```python
from build123d import *

# Parameters (mm, degrees)
BOSS_EXTRUDE1_DEPTH = 3.175
SKETCH2_R           = 2.159
CUT_EXTRUDE1_DEPTH  = 38.162422217
CUT_EXTRUDE2_DEPTH  = 38.162422217
FILLET1_R           = 6.35
FILLET2_R           = 1.905


with BuildPart() as part:
    # Sketch1 → Boss-Extrude1 (new body)
    with BuildSketch(Plane(origin=(0, 0, 0), x_dir=(1, 0, 0), z_dir=(0, 1, 0))):
        Polygon((-17.4625, 31.75), (0, 22.225), (17.4625, 31.75), (19.05, 3.175), (0, -19.05), (-19.05, 3.175), align=None)
    extrude(amount=BOSS_EXTRUDE1_DEPTH)

    # Sketch2 → Cut-Extrude1 (cut, through all)
    with BuildSketch(Plane(origin=(0, 3.175, 0), x_dir=(1, 0, 0), z_dir=(0, 1, 0))):
        with Locations(Location((0, -10.4775, 0), (0, 0, 270))):
            Circle(SKETCH2_R)
        with Locations(Location((-12.7, 3.4925, 0), (0, 0, 270))):
            Circle(SKETCH2_R)
        with Locations(Location((12.7, 3.4925, 0), (0, 0, 270))):
            Circle(SKETCH2_R)
        with Locations(Location((-12.7, 22.5425, 0), (0, 0, 270))):
            Circle(SKETCH2_R)
        with Locations(Location((12.7, 22.5425, 0), (0, 0, 270))):
            Circle(SKETCH2_R)
    extrude(amount=-CUT_EXTRUDE1_DEPTH, mode=Mode.SUBTRACT)

    # Sketch3 → Cut-Extrude2 (cut, through all)
    with BuildSketch(Plane(origin=(0, 3.175, 0), x_dir=(1, 0, 0), z_dir=(0, 1, 0))):
        Polygon((-9.366701395, 17.207620695), (-9.975545431, 6.248428041), (0, -5.389708296), (9.975545431, 6.248428041), (9.366701395, 17.207620695), (0, 12.098510843), align=None)
    extrude(amount=-CUT_EXTRUDE2_DEPTH, mode=Mode.SUBTRACT)

    # Fillet1
    fillet1_edges = [part.edges().sort_by_distance(p)[0] for p in [
        (-17.4625, 1.5875, -31.75),
        (0, 1.5875, -22.225),
        (17.4625, 1.5875, -31.75),
        (19.05, 1.5875, -3.175),
        (0, 1.5875, 19.05),
        (-19.05, 1.5875, -3.175),
    ]]
    fillet(fillet1_edges, radius=FILLET1_R)

    # Fillet2
    fillet2_edges = [part.edges().sort_by_distance(p)[0] for p in [
        (-9.366701395, 1.5875, -17.207620695),
        (0, 1.5875, -12.098510843),
        (9.366701395, 1.5875, -17.207620695),
        (9.975545431, 1.5875, -6.248428041),
        (0, 1.5875, 5.389708296),
        (-9.975545431, 1.5875, -6.248428041),
    ]]
    fillet(fillet2_edges, radius=FILLET2_R)


solid = part.part
```
Work out the finished part from the listing and answer in its coordinate system (mm). A direction names the side the tool comes from. Coordinates: 2 decimals unless noted, no trailing zeros. Loops run counter-clockwise (first coordinate to the right, second up) from the corner with the lowest first, then second, coordinate; pieces in that order, holes last.
1) Section C-C (z = -22.5) is taken. Give the vertices of the cut face in (x, y) (3 decimals), plus the area to 3 significant figures.
Results:
outline: (-17.927, 0) - (-14.859, 0) - (-14.859, 3.175) - (-17.927, 3.175) - close; (-10.541, 0) - (10.541, 0) - (10.541, 3.175) - (-10.541, 3.175) - close; (14.859, 0) - (17.927, 0) - (17.927, 3.175) - (14.859, 3.175) - close
area: 86.4 mm2
2) For a pull along Z with two mould halves and no side action, classify faces 4 (the flat face through (18.46, 1.57, -13.83)), 5 (the cylindrical face through (10.785, 1.61, -2.496)), 6 (the cylindrical face through (-0.077, 1.61, 15.642)) as +Z half, -Z half, draft (parallel to the pull), parting line (faces both ways), or undercut.
Results:
face 4: -Z half
face 5: undercut
face 6: +Z half
3) Section A-A (x = 0) is taken. Give the vertices of the cut face in (y, z) (1 decimal).
Results:
outline: (0, -23.1) - (3.2, -23.1) - (3.2, -12.4) - (0, -12.4) - close; (0, 4.4) - (3.2, 4.4) - (3.2, 8.3) - (0, 8.3) - close; (0, 12.6) - (3.2, 12.6) - (3.2, 15.6) - (0, 15.6) - close
4) Consider probe 1 along Z at (x, y) = (-14, 3); probe 2 along Z at (x, y) = (-14.5, 2.45); probe 3 along X at (y, z) = (0.7, -2.5). Determine where each line is inside the solid, lowest interval first.
Results:
probe 1: z = -27.27 to -24.27, -20.82 to -5.22, -1.77 to 2.72
probe 2: z = -27.05 to -23.73, -21.35 to -4.68, -2.3 to 2.13
probe 3: x = -18.23 to -14.62, -10.78 to -6.76, 6.76 to 10.78, 14.62 to 18.23
5) Section D-D (x = 7.5) is taken. Give the vertices of the cut face in (y, z) (3 decimals), plus the area to 3 significant figures.
Results:
outline: (0, -26.316) - (3.175, -26.316) - (3.175, -15.992) - (0, -15.992) - close; (0, -3.36) - (3.175, -3.36) - (3.175, 10.3) - (0, 10.3) - close
area: 76.2 mm2
6) For faces 1 (the cylindrical face through (-0.013, 1.565, -12.364)), 2 (the flat face through (11.193, 1.565, 5.991)), 3 (the flat face through (-5.88, 1.57, -25.43)), determine the directions among +Z, -Z, +X, -X, +Y, -Y from which every point of the face is accessible in a straight line to the end or side of a thin tool.
Results:
face 1: +Y, -Y
face 2: +Z, +X, +Y, -Y
face 3: -Z, +Y, -Y
7) Flat-ended cylindrical pins translate along their axes: pin 1 (1.5 mm diameter, centred on x = 9, y = 1.5, fed in from +Z) (3 decimals); pin 2 (1 mm diameter, centred on y = 2, z = -9, fed in from +X); pin 3 (1.5 mm diameter, centred on y = 2, z = -10, fed in from +X). Find the tip coordinate at first contact, or state that the pin passes through.
Results:
pin 1: stops at z = 9.425
pin 2: stops at x = 18.75
pin 3: stops at x = 18.71
8) Section B-B (y = 1.5) is taken. Give the number of separate pieces and of enclosed holes in the cut face, plus the area to 3 significant figures.
Results:
separate pieces: 1
enclosed holes: 6
area: 894 mm2
